Source: CAD feature listing. Evaluate the final solid. Frame: model axes, mm. Face numbers are marked on the shaded views. A direction names the side the tool comes from. Give positions to 0.01 mm unless a question says otherwise; leave off trailing zeros. Order: outer loops, then holes, each group sorted by start corner. A loop starts at its lowest first (then second) coordinate and runs counter-clockwise, first axis right, second up. Notation, with made-up numbers: (18, 84) - (54, 84) arc R12 cw to (54, 100) - close; hole circle Ø4 at (-3, -18). An arc over 180 degrees is marked (long way). One line per item, written item: value. Start each with the question number.
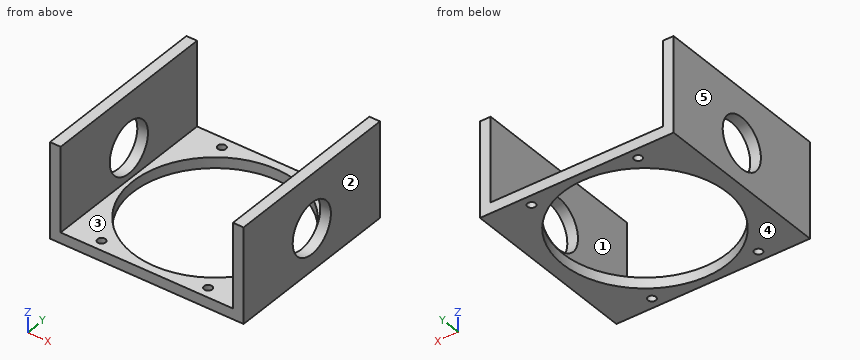
from build123d import *

# Parameters (mm, degrees)
BOSS_EXTRUDE2_DEPTH      = 51
BOSS_EXTRUDE2_DEPTH_BACK = 51
SKETCH4_R                = 46.25
SKETCH4_R_2              = 2.25
CUT_EXTRUDE1_DEPTH       = 89.519630491
SKETCH5_R                = 14.2875
CUT_EXTRUDE2_DEPTH       = 125.024191189


with BuildPart() as part:
    # Sketch3 → Boss-Extrude2 (new, two sides: drawn at the far end of the back side and taken through both)
    with BuildSketch(Plane(origin=(0, 0, 0), x_dir=(1, 0, 0), z_dir=(0, 1, 0)).offset(-BOSS_EXTRUDE2_DEPTH_BACK)):
        Polygon((-48.5, -30), (-54.5, -30), (-54.5, 23.5865), (54.5, 23.5865), (54.5, -30), (48.5, -30), (48.5, 17.5865), (-48.5, 17.5865), align=None)
    extrude(amount=BOSS_EXTRUDE2_DEPTH + BOSS_EXTRUDE2_DEPTH_BACK)

    # Sketch4 → Cut-Extrude1 (cut, through all)
    with BuildSketch(Plane.XY.offset(-17.5865)):
        Circle(SKETCH4_R)
        with Locations((-30, 45)):
            Circle(SKETCH4_R_2)
        with Locations((30, 45)):
            Circle(SKETCH4_R_2)
        with Locations((30, -45)):
            Circle(SKETCH4_R_2)
        with Locations((-30, -45)):
            Circle(SKETCH4_R_2)
    extrude(amount=-CUT_EXTRUDE1_DEPTH, mode=Mode.SUBTRACT)

    # Sketch5 → Cut-Extrude2 (cut, through all)
    with BuildSketch(Plane(origin=(54.5, 0, 0), x_dir=(0, 0, -1), z_dir=(1, 0, 0))):
        Circle(SKETCH5_R)
    extrude(amount=-CUT_EXTRUDE2_DEPTH, mode=Mode.SUBTRACT)


solid = part.part
1. Ray query, L1, parallel to X at y = -37, z = -4; L2, parallel to Y at x = 30, z = -20.15; L3, parallel to Y at x = -50.7, z = 0. Return the intervals inside material, ascending.
2. Contact query for flat-ended pins moving along their axis: pin 1 Ø4 at (x, y) = (-42.5, 36.5) entering from +Z; pin 2 Ø3.5 at (x, y) = (30, -45) entering from -Z. Output: stop coordinate, or through.
3. Section A-A on y = 0. Return the cut outline in (x, z).
4. Draft query along X for the marked faces 3, 4 and 5. Return one class per face: pulls with the +X half, pulls with the -X half, needs draft (parallel to the pull), parting line crosses it, or undercut.
5. Section B-B on x = 0. Return the cut outline in (y, z), then the cut area to 3 significant figures.
6. Section C-C on z = 0. Return the cut outline in (x, y).
7. Section D-D on z = -19. Return the cut outline in (x, y), then the cut area to 3 significant figures.
8. Set-up query: the marked faces 1 and 2. Return all of +Z, -Z, +X, -X, +Y, -Y with unobstructed straight access to the full face (end or side cutting, diameter ignored); none if empty.
Data:
1. L1: x = -54.5 to -48.5, 48.5 to 54.5
1. L2: y = -51 to -47.25, -42.75 to -35.2, 35.2 to 42.75, 47.25 to 51
1. L3: y = -51 to -14.29, 14.29 to 51
2. pin 1: stops at z = -17.59
2. pin 2: passes through
3. outline: (-54.5, -23.59) - (-46.25, -23.59) - (-46.25, -17.59) - (-48.5, -17.59) - (-48.5, -14.29) - (-54.5, -14.29) - close; (-54.5, 14.29) - (-48.5, 14.29) - (-48.5, 30) - (-54.5, 30) - close; (46.25, -23.59) - (54.5, -23.59) - (54.5, -14.29) - (48.5, -14.29) - (48.5, -17.59) - (46.25, -17.59) - close; (48.5, 14.29) - (54.5, 14.29) - (54.5, 30) - (48.5, 30) - close
4. face 3: undercut
4. face 4: needs draft
4. face 5: pulls with the -X half
5. outline: (-51, -23.59) - (-46.25, -23.59) - (-46.25, -17.59) - (-51, -17.59) - close; (46.25, -23.59) - (51, -23.59) - (51, -17.59) - (46.25, -17.59) - close
5. area: 57.0 mm2
6. outline: (-54.5, -51) - (-48.5, -51) - (-48.5, -14.29) - (-54.5, -14.29) - close; (-54.5, 14.29) - (-48.5, 14.29) - (-48.5, 51) - (-54.5, 51) - close; (48.5, -51) - (54.5, -51) - (54.5, -14.29) - (48.5, -14.29) - close; (48.5, 14.29) - (54.5, 14.29) - (54.5, 51) - (48.5, 51) - close
7. outline: (-54.5, -51) - (54.5, -51) - (54.5, 51) - (-54.5, 51) - close; hole circle Ø92.5 at (0, 0); hole circle Ø4.5 at (-30, -45); hole circle Ø4.5 at (-30, 45); hole circle Ø4.5 at (30, -45); hole circle Ø4.5 at (30, 45)
7. area: 4,330 mm2
8. face 1: +Z, +Y, -Y
8. face 2: +Z, -Z, +X, +Y, -Y
